```python
from build123d import *

# Parameters (mm, degrees)
BOX193_W          = 10
BOX193_H          = 2
BOX193_DEPTH      = 1.5
CYLINDER075_R     = 1.6
CYLINDER075_DEPTH = 2
BOX191_W          = 10
BOX191_H          = 2
BOX191_DEPTH      = 9
FILLET044_R       = 3


with BuildPart() as cube182:
    # Box193 → Box193 (new body)
    with BuildSketch(Plane(origin=(54, 15, -2.5), x_dir=(1, 0, 0), z_dir=(0, 0, 1))):
        with Locations((5, 1)):
            Rectangle(BOX193_W, BOX193_H)
    extrude(amount=BOX193_DEPTH)


with BuildPart() as cylinder156:
    # Cylinder075 → Cylinder075 (new body)
    with BuildSketch(Plane(origin=(59, 15, -7), x_dir=(1, 0, 0), z_dir=(0, -1, 0))):
        Circle(CYLINDER075_R)
    extrude(amount=CYLINDER075_DEPTH)


with BuildPart() as fusion060:
    # Box191 → Box191 (new body)
    with BuildSketch(Plane(origin=(54, 13, -10), x_dir=(1, 0, 0), z_dir=(0, 0, 1))):
        with Locations((5, 1)):
            Rectangle(BOX191_W, BOX191_H)
    extrude(amount=BOX191_DEPTH)

    # Fillet044
    fillet044_edges = [fusion060.edges().sort_by_distance(p)[0] for p in [
        (54, 14, -10),
        (64, 14, -10),
    ]]
    fillet(fillet044_edges, radius=FILLET044_R)

    # Cut099: cut Cylinder156
    add(cylinder156.part, mode=Mode.SUBTRACT)

    # Fusion060: union Cube182
    add(cube182.part)


solid = fusion060.part
```
Could you check a few things on this model? Use its own coordinates, in mm. A direction names the side the tool comes from. Coordinates: 2 decimals unless noted, no trailing zeros. Write each loop counter-clockwise with the first axis right and the second up, starting at its lowest first coordinate (ties: lowest second). Pieces come first, ordered by that corner, then holes. Notation, with made-up numbers: M 23,48 L 47,48 A32 cw 47,80 Z; hole C -18.75,65 d8. An arc over 180 degrees is marked long. Answer as CSV lines item,"result". Start each with the question number.
1) I want a section at C-C, the plane z = -6. Please give me the cut outline in (x, y), and give its area (3 significant figures).
2) I want a section at B-B, the plane y = 13.8. Please give me the cut outline in (x, z).
3) I want a section at D-D, the plane y = 15.95. Please give me the cut outline in (x, z).
4) We'd pull the mould along Z, two halves only. Please class faces 1 (the cylindrical face through (60.48, 14.01, -7.61)), 2 (the flat face through (59, 16, -2.5)), 3 (the flat face through (59, 15, -1)), 4 (the flat face through (59, 13, -5)): +Z half, -Z half, draft (parallel to the pull), parting line (faces both ways), or undercut.
5) For P1, Ø1.5, axis at x = 56.5, z = -6.5, coming from the +Y side; P2, Ø1.6, axis at x = 58.5, y = 16, coming from the -Z side, each with a flat end and sliding along its axis, tell me the tip position at first contact or that it passes through.
6) Please list where these lines run through material, in increasing order: line 1 (Z direction, x = 59, y = 14.35); line 2 (Y direction, x = 61.25, z = -7.75); line 3 (X direction, y = 13.4, z = -7.5). Write a range as from..to.
7) I want a section at A-A, the plane x = 59. Please give me the cut outline in (y, z), and give its area (3 significant figures).
8) For faces 5 (the flat face through (60, 15, -5)), 6 (the flat face through (59, 17, -2)), which set-ups out of +Z, -Z, +X, -X, +Y, -Y let a thin tool reach every point of the face, with its end or its side?
Data:
1,outline,"M 54,13 L 57.75,13 L 57.75,15 L 54,15 Z; M 60.25,13 L 64,13 L 64,15 L 60.25,15 Z"
1,area,"15.0 mm^2"
2,outline,"M 54,-7 A3 ccw 57,-10 L 61,-10 A3 ccw 64,-7 L 64,-1 L 54,-1 Z; hole C 59,-7 d3.2"
3,outline,"M 54,-2.5 L 64,-2.5 L 64,-1 L 54,-1 Z"
4,face 1,"undercut"
4,face 2,"-Z half"
4,face 3,"+Z half"
4,face 4,"draft"
5,P1,"stops at y = 15"
5,P2,"stops at z = -2.5"
6,line 1,"z = -10..-8.6, -5.4..-1"
6,line 2,"y = 13..15"
6,line 3,"x = 54.04..57.48, 60.52..63.96"
7,outline,"M 13,-10 L 15,-10 L 15,-8.6 L 13,-8.6 Z; M 13,-5.4 L 15,-5.4 L 15,-2.5 L 17,-2.5 L 17,-1 L 13,-1 Z"
7,area,"14.6 mm^2"
8,face 5,"-Z, +X, -X, +Y"
8,face 6,"+Z, -Z, +X, -X, +Y"
